Here's how the part is built. I have some questions about the finished solid (model axes, mm). Round coordinates to 2 decimals unless told otherwise and drop trailing zeros. Loops run counter-clockwise (first coordinate to the right, second up) from the corner with the lowest first, then second, coordinate; pieces in that order, holes last. Notation, with made-up numbers: M 16,71 L 33,71 A24 ccw 33,95 Z; hole C -6.5,88.5 d2. An arc over 180 degrees is marked long. Answer as a JSON object with one key per item and string values.
from build123d import *

# Parameters (mm, degrees)
F0_W     = 125
F0_H     = 12
F1_DEPTH = 5
F2_W     = 120
F2_H     = 9.5
F3_DEPTH = 1
F4_R     = 2.5887659848
F5_DEPTH = 5
F5_TAPER = 20


with BuildPart() as f1:
    # F0 (on Top) → F1 (new body)
    with BuildSketch(Plane.XY):
        with Locations((62.5, 6)):
            Rectangle(F0_W, F0_H)
    extrude(amount=F1_DEPTH)

    # F2 (on face) → F3 (cut)
    with BuildSketch(Plane.XY.offset(5)):
        with Locations((63, 5.95)):
            Rectangle(F2_W, F2_H)
    extrude(amount=-F3_DEPTH, mode=Mode.SUBTRACT)

    # F4 (on face) → F5 (cut)
    with BuildSketch(Plane(origin=(0, 0, 0), x_dir=(1, 0, 0), z_dir=(0, 0, -1))):
        with Locations((6.7181466147, -6.0111363418)):
            Circle(F4_R)
        with Locations((32.7181466147, -6.0111363418)):
            Circle(F4_R)
        with Locations((58.7181466147, -6.0111363418)):
            Circle(F4_R)
        with Locations((84.7181466147, -6.0111363418)):
            Circle(F4_R)
        with Locations((110.7181466147, -6.0111363418)):
            Circle(F4_R)
    extrude(amount=-F5_DEPTH, taper=F5_TAPER, mode=Mode.SUBTRACT)


solid = f1.part
Item 1: Please list where these lines run through material, in increasing order: probe 1 along X at (y, z) = (7, 3.5); probe 2 along X at (y, z) = (7, 2.3); probe 3 along Y at (x, z) = (116, 4.6). Write a range as from..to.
Resolved:
{"probe 1": "0..5.85, 7.58..31.85, 33.58..57.85, 59.58..83.85, 85.58..109.85, 111.58..125", "probe 2": "0..5.27, 8.16..31.27, 34.16..57.27, 60.16..83.27, 86.16..109.27, 112.16..125", "probe 3": "0..1.2, 10.7..12"}
Item 2: I'm going to push flat-ended pins straight in: pin 1 Ø1 at (x, y) = (98.5, 4) entering from +Z; pin 2 Ø0.5 at (x, z) = (52, 4.5) entering from -Y. Where does each tip first touch, or does it pass through?
Resolved:
{"pin 1": "z = 4", "pin 2": "y = 0"}
Item 3: I want a section at A-A, the plane x = 14.5. Please give me the cut outline in (y, z).
Resolved:
{"outline": "M 0,0 L 12,0 L 12,5 L 10.7,5 L 10.7,4 L 1.2,4 L 1.2,5 L 0,5 Z"}
Item 4: I want a section at B-B, the plane z = 2. Please give me the cut outline in (x, y), then the cut area to 3 significant figures.
Resolved:
{"outline": "M 0,0 L 125,0 L 125,12 L 0,12 Z; hole C 6.72,6.01 d3.72; hole C 32.72,6.01 d3.72; hole C 58.72,6.01 d3.72; hole C 84.72,6.01 d3.72; hole C 110.72,6.01 d3.72", "area": "1,450 mm²"}
Item 5: If we mould it in two halves opening along X, with no side actions, what happens to faces 1 (the face through (62, 6, 4)), 2 (the face through (62, 6, 0)), 3 (the face through (0, 6, 2))? For each: pulls with the +X half, pulls with the -X half, needs draft (parallel to the pull), parting line crosses it, or undercut.
Resolved:
{"face 1": "undercut", "face 2": "needs draft", "face 3": "pulls with the -X half"}
